```python
from build123d import *

# Parameters (mm, degrees)
SKETCH_1_R      = 1.5
EXTRUDE_1_DEPTH = 3


with BuildPart() as part:
    # 草图1 → 凸台-拉伸1 (new body)
    with BuildSketch(Plane.XY):
        with BuildLine():
            ThreePointArc((-6.655206862, 1.127262893), (-6.156247128, 0.795666927), (-5.592723466, 0.592300797))
            ThreePointArc((-5.592723466, 0.592300797), (-5.612902321, 0.353133882), (-5.622858145, 0.113323788))
            ThreePointArc((-5.622858145, 0.113323788), (-6.207426789, -0.017810496), (-6.744012071, -0.284255492))
            ThreePointArc((-6.744012071, -0.284255492), (-6.736680417, -0.423836007), (-6.726460182, -0.563234787))
            ThreePointArc((-6.726460182, -0.563234787), (-6.160711622, -0.760326816), (-5.564316992, -0.81716119))
            ThreePointArc((-5.564316992, -0.81716119), (-5.524383498, -1.053832513), (-5.474388197, -1.288584444))
            ThreePointArc((-5.474388197, -1.288584444), (-6.007979772, -1.560975215), (-6.461445064, -1.952492684))
            ThreePointArc((-6.461445064, -1.952492684), (-6.419631485, -2.085864712), (-6.37506527, -2.218342354))
            ThreePointArc((-6.37506527, -2.218342354), (-5.778075948, -2.26854643), (-5.186284018, -2.175277933))
            ThreePointArc((-5.186284018, -2.175277933), (-5.088747343, -2.394582736), (-4.981942305, -2.609526178))
            ThreePointArc((-4.981942305, -2.609526178), (-5.431029289, -3.006058119), (-5.772881701, -3.49804758))
            ThreePointArc((-5.772881701, -3.49804758), (-5.699213497, -3.616830866), (-5.623101562, -3.734063313))
            ThreePointArc((-5.623101562, -3.734063313), (-5.032382511, -3.634224927), (-4.482377745, -3.396713964))
            ThreePointArc((-4.482377745, -3.396713964), (-4.333366477, -3.584872518), (-4.176462656, -3.766501784))
            ThreePointArc((-4.176462656, -3.766501784), (-4.512827263, -4.262259337), (-4.721586948, -4.823807282))
            ThreePointArc((-4.721586948, -4.823807282), (-4.620692965, -4.920538235), (-4.517817702, -5.01515934))
            ThreePointArc((-4.517817702, -5.01515934), (-3.970485973, -4.771551707), (-3.496827193, -4.404721964))
            ThreePointArc((-3.496827193, -4.404721964), (-3.305704259, -4.549911576), (-3.108560498, -4.686814231))
            ThreePointArc((-3.108560498, -4.686814231), (-3.311067702, -5.250647125), (-3.373617523, -5.846469431))
            ThreePointArc((-3.373617523, -5.846469431), (-3.2518373, -5.91507009), (-3.128662741, -5.981134462))
            ThreePointArc((-3.128662741, -5.981134462), (-2.6591092, -5.609064345), (-2.291558128, -5.135965084))
            ThreePointArc((-2.291558128, -5.135965084), (-2.070332484, -5.229062957), (-1.845336051, -5.312636903))
            ThreePointArc((-1.845336051, -5.312636903), (-1.901261581, -5.909117443), (-1.813671302, -6.501776404))
            ThreePointArc((-1.813671302, -6.501776404), (-1.678656738, -6.537936338), (-1.542922393, -6.571292908))
            ThreePointArc((-1.542922393, -6.571292908), (-1.180650815, -6.094138841), (-0.942302038, -5.544496629))
            ThreePointArc((-0.942302038, -5.544496629), (-0.704874106, -5.57965308), (-0.466162354, -5.604647059))
            ThreePointArc((-0.466162354, -5.604647059), (-0.371992202, -6.196296181), (-0.139765443, -6.748552854))
            ThreePointArc((-0.139765443, -6.748552854), (0, -6.75), (0.139765443, -6.748552854))
            ThreePointArc((0.139765443, -6.748552854), (0.371992202, -6.196296181), (0.466162354, -5.604647059))
            ThreePointArc((0.466162354, -5.604647059), (0.704874106, -5.57965308), (0.942302038, -5.544496629))
            ThreePointArc((0.942302038, -5.544496629), (1.180650815, -6.094138841), (1.542922393, -6.571292908))
            ThreePointArc((1.542922393, -6.571292908), (1.678656738, -6.537936338), (1.813671302, -6.501776404))
            ThreePointArc((1.813671302, -6.501776404), (1.901261581, -5.909117443), (1.845336051, -5.312636903))
            ThreePointArc((1.845336051, -5.312636903), (2.070332484, -5.229062957), (2.291558128, -5.135965084))
            ThreePointArc((2.291558128, -5.135965084), (2.6591092, -5.609064345), (3.128662741, -5.981134462))
            ThreePointArc((3.128662741, -5.981134462), (3.2518373, -5.91507009), (3.373617523, -5.846469431))
            ThreePointArc((3.373617523, -5.846469431), (3.311067702, -5.250647125), (3.108560498, -4.686814231))
            ThreePointArc((3.108560498, -4.686814231), (3.305704259, -4.549911576), (3.496827193, -4.404721964))
            ThreePointArc((3.496827193, -4.404721964), (3.970485973, -4.771551707), (4.517817702, -5.01515934))
            ThreePointArc((4.517817702, -5.01515934), (4.620692965, -4.920538235), (4.721586948, -4.823807282))
            ThreePointArc((4.721586948, -4.823807282), (4.512827263, -4.262259337), (4.176462656, -3.766501784))
            ThreePointArc((4.176462656, -3.766501784), (4.333366477, -3.584872518), (4.482377745, -3.396713964))
            ThreePointArc((4.482377745, -3.396713964), (5.032382511, -3.634224927), (5.623101562, -3.734063313))
            ThreePointArc((5.623101562, -3.734063313), (5.699213497, -3.616830866), (5.772881701, -3.49804758))
            ThreePointArc((5.772881701, -3.49804758), (5.431029289, -3.006058119), (4.981942305, -2.609526178))
            ThreePointArc((4.981942305, -2.609526178), (5.088747343, -2.394582736), (5.186284018, -2.175277933))
            ThreePointArc((5.186284018, -2.175277933), (5.778075948, -2.26854643), (6.37506527, -2.218342354))
            ThreePointArc((6.37506527, -2.218342354), (6.419631485, -2.085864712), (6.461445064, -1.952492684))
            ThreePointArc((6.461445064, -1.952492684), (6.007979772, -1.560975215), (5.474388197, -1.288584444))
            ThreePointArc((5.474388197, -1.288584444), (5.524383498, -1.053832513), (5.564316992, -0.81716119))
            ThreePointArc((5.564316992, -0.81716119), (6.160711622, -0.760326816), (6.726460182, -0.563234787))
            ThreePointArc((6.726460182, -0.563234787), (6.736680417, -0.423836007), (6.744012071, -0.284255492))
            ThreePointArc((6.744012071, -0.284255492), (6.207426789, -0.017810496), (5.622858145, 0.113323788))
            ThreePointArc((5.622858145, 0.113323788), (5.612902321, 0.353133882), (5.592723466, 0.592300797))
            ThreePointArc((5.592723466, 0.592300797), (6.156247128, 0.795666927), (6.655206862, 1.127262893))
            ThreePointArc((6.655206862, 1.127262893), (6.630438942, 1.264823873), (6.602827997, 1.401842518))
            ThreePointArc((6.602827997, 1.401842518), (6.016838352, 1.526473321), (5.418023237, 1.508111471))
            ThreePointArc((5.418023237, 1.508111471), (5.348741848, 1.737911576), (5.269718556, 1.964546346))
            ThreePointArc((5.269718556, 1.964546346), (5.764962986, 2.301665991), (6.165782418, 2.7469305))
            ThreePointArc((6.165782418, 2.7469305), (6.107582604, 2.874010218), (6.046763956, 2.999857607))
            ThreePointArc((6.046763956, 2.999857607), (5.448189833, 2.974843206), (4.872754002, 2.808138963))
            ThreePointArc((4.872754002, 2.808138963), (4.748500253, 3.013489895), (4.615597848, 3.213352223))
            ThreePointArc((4.615597848, 3.213352223), (5.011445017, 3.663042916), (5.28893919, 4.193998361))
            ThreePointArc((5.28893919, 4.193998361), (5.200964389, 4.302611931), (5.110759497, 4.40938061))
            ThreePointArc((5.110759497, 4.40938061), (4.53721151, 4.236292751), (4.021311713, 3.931720757))
            ThreePointArc((4.021311713, 3.931720757), (3.849892924, 4.099719561), (3.671462152, 4.260251362))
            ThreePointArc((3.671462152, 4.260251362), (3.943039527, 4.794257382), (4.07977246, 5.37754188))
            ThreePointArc((4.07977246, 5.37754188), (3.967550453, 5.460864712), (3.853627223, 5.541846012))
            ThreePointArc((3.853627223, 5.541846012), (3.341143501, 5.231560443), (2.917195619, 4.808258075))
            ThreePointArc((2.917195619, 4.808258075), (2.709382663, 4.928348769), (2.496634987, 5.039463239))
            ThreePointArc((2.496634987, 5.039463239), (2.626878362, 5.624231026), (2.614258623, 6.223194666))
            ThreePointArc((2.614258623, 6.223194666), (2.484840731, 6.27599128), (2.354357378, 6.326096848))
            ThreePointArc((2.354357378, 6.326096848), (1.935139158, 5.898109951), (1.629781396, 5.382674856))
            ThreePointArc((1.629781396, 5.382674856), (1.398631925, 5.447311698), (1.164935063, 5.502027108))
            ThreePointArc((1.164935063, 5.502027108), (1.145660769, 6.100813549), (0.984481302, 6.677821244))
            ThreePointArc((0.984481302, 6.677821244), (0.845999327, 6.696774234), (0.7071546, 6.712855754))
            ThreePointArc((0.7071546, 6.712855754), (0.407542904, 6.19405952), (0.239962014, 5.618878378))
            ThreePointArc((0.239962014, 5.618878378), (0, 5.624), (-0.239962014, 5.618878378))
            ThreePointArc((-0.239962014, 5.618878378), (-0.407542904, 6.19405952), (-0.7071546, 6.712855754))
            ThreePointArc((-0.7071546, 6.712855754), (-0.845999327, 6.696774234), (-0.984481302, 6.677821244))
            ThreePointArc((-0.984481302, 6.677821244), (-1.145660769, 6.100813549), (-1.164935063, 5.502027108))
            ThreePointArc((-1.164935063, 5.502027108), (-1.398631925, 5.447311698), (-1.629781396, 5.382674855))
            ThreePointArc((-1.629781396, 5.382674855), (-1.935139158, 5.898109951), (-2.354357378, 6.326096848))
            ThreePointArc((-2.354357378, 6.326096848), (-2.484840731, 6.27599128), (-2.614258623, 6.223194666))
            ThreePointArc((-2.614258623, 6.223194666), (-2.626878362, 5.624231026), (-2.496634987, 5.039463239))
            ThreePointArc((-2.496634987, 5.039463239), (-2.709382663, 4.928348769), (-2.917195619, 4.808258075))
            ThreePointArc((-2.917195619, 4.808258075), (-3.341143501, 5.231560443), (-3.853627223, 5.541846012))
            ThreePointArc((-3.853627223, 5.541846012), (-3.967550453, 5.460864712), (-4.07977246, 5.37754188))
            ThreePointArc((-4.07977246, 5.37754188), (-3.943039527, 4.794257382), (-3.671462152, 4.260251362))
            ThreePointArc((-3.671462152, 4.260251362), (-3.849892924, 4.099719561), (-4.021311713, 3.931720757))
            ThreePointArc((-4.021311713, 3.931720757), (-4.53721151, 4.236292751), (-5.110759497, 4.40938061))
            ThreePointArc((-5.110759497, 4.40938061), (-5.200964389, 4.302611931), (-5.28893919, 4.193998361))
            ThreePointArc((-5.28893919, 4.193998361), (-5.011445017, 3.663042916), (-4.615597848, 3.213352223))
            ThreePointArc((-4.615597848, 3.213352223), (-4.748500253, 3.013489895), (-4.872754002, 2.808138963))
            ThreePointArc((-4.872754002, 2.808138963), (-5.448189833, 2.974843206), (-6.046763956, 2.999857607))
            ThreePointArc((-6.046763956, 2.999857607), (-6.107582604, 2.874010218), (-6.165782418, 2.7469305))
            ThreePointArc((-6.165782418, 2.7469305), (-5.764962986, 2.301665991), (-5.269718556, 1.964546346))
            ThreePointArc((-5.269718556, 1.964546346), (-5.348741848, 1.737911576), (-5.418023237, 1.508111471))
            ThreePointArc((-5.418023237, 1.508111471), (-6.016838352, 1.526473321), (-6.602827997, 1.401842518))
            ThreePointArc((-6.602827997, 1.401842518), (-6.630438942, 1.264823873), (-6.655206862, 1.127262893))
        make_face()
        Circle(SKETCH_1_R, mode=Mode.SUBTRACT)
    extrude(amount=EXTRUDE_1_DEPTH)


solid = part.part
```
Here's how the part is built. I have some questions about the finished solid (model axes, mm). A direction names the side the tool comes from. Coordinates: 2 decimals unless noted, no trailing zeros. Order: outer loops, then holes, each group sorted by start corner. A loop starts at its lowest first (then second) coordinate and runs counter-clockwise, first axis right, second up. Notation, with made-up numbers: (-1.5, 0) - (24.5, 0) arc R21 cw to (24.5, 32) - close; hole circle Ø9 at (-3.5, 86.25). An arc over 180 degrees is marked (long way). One line per question, with ' | ' between items.
(1) Will these pins go through, and if not, where does the flat tip stop? pin 1 (1 mm diameter, centred on x = -4, z = 0.5, fed in from +Y); pin 2 (1.5 mm diameter, centred on y = 4, z = 0.5, fed in from -X).
Report:
pin 1: stops at y = 5.54 | pin 2: stops at x = -5.29
(2) For faces 1 (the cylindrical face through (6.215, -0.021, 1.479)), 2 (the cylindrical face through (-0.404, 6.186, 1.479)), 3 (the cylindrical face through (5.02, -3.63, 1.48)), 4 (the cylindrical face through (-2.67, -5.62, 1.48)), which set-ups out of +Z, -Z, +X, -X, +Y, -Y let a thin tool reach every point of the face, with its end or its side?
Report:
face 1: +Z, -Z, +X | face 2: +Z, -Z, +Y | face 3: +Z, -Z | face 4: +Z, -Z, -Y
(3) Suppose I cut it at B-B on y = 6. List the corners of the cut face in (x, z) for me, and give its area (3 significant figures).
Report:
outline: (-2.64, 0) - (-2.02, 0) - (-2.02, 3) - (-2.64, 3) - close; (-1.16, 0) - (-0.33, 0) - (-0.33, 3) - (-1.16, 3) - close; (0.33, 0) - (1.16, 0) - (1.16, 3) - (0.33, 3) - close; (2.02, 0) - (2.64, 0) - (2.64, 3) - (2.02, 3) - close | area: 8.66 mm2
(4) Suppose I cut it at A-A on y = 0.75. List the corners of the cut face in (x, z) for me.
Report:
outline: (-6.06, 0) - (-1.3, 0) - (-1.3, 3) - (-6.06, 3) - close; (1.3, 0) - (6.06, 0) - (6.06, 3) - (1.3, 3) - close
(5) If I drill on L1, parallel to Y at x = 0, z = 1.4; L2, parallel to X at y = 5, z = 0.2; L3, parallel to Y at x = -1.25, z = 2.7, over which ranges is the centre line in solid material (lowest first)?
Report:
L1: y = -6.75 to -1.5, 1.5 to 5.62 | L2: x = -4.01 to -3.08, -2.57 to 2.57, 3.08 to 4.01 | L3: y = -6.21 to -0.83, 0.83 to 5.48
(6) If we mould it in two halves opening along X, with no side actions, what happens to faces 5 (the flat face through (-2, 0, 0)), 6 (the cylindrical face through (5.456, 2.976, 1.479)), 7 (the cylindrical face through (-6.001, -1.556, 1.479))? For each: pulls with the +X half, pulls with the -X half, needs draft (parallel to the pull), parting line crosses it, or undercut.
Report:
face 5: needs draft | face 6: undercut | face 7: pulls with the -X half
